from build123d import *

# Parameters (mm, degrees)
SKETCH1_W           = 43
SKETCH1_H           = 43
BOSS_EXTRUDE1_DEPTH = 47
SKETCH2_R           = 10.75
BOSS_EXTRUDE2_DEPTH = 1
SKETCH3_R           = 2.5
BOSS_EXTRUDE3_DEPTH = 20
CHAMFER1_SIZE       = 3
SKETCH4_R           = 1.75
CUT_EXTRUDE2_DEPTH  = 10


with BuildPart() as part:
    # Sketch1 → Boss-Extrude1 (new body)
    with BuildSketch(Plane(origin=(0, 0, 0), x_dir=(1, 0, 0), z_dir=(0, 1, 0))):
        with Locations((21.5, 21.5)):
            Rectangle(SKETCH1_W, SKETCH1_H)
    extrude(amount=BOSS_EXTRUDE1_DEPTH)

    # Sketch2 → Boss-Extrude2 (add)
    with BuildSketch(Plane(origin=(0, 47, 0), x_dir=(1, 0, 0), z_dir=(0, 1, 0))):
        with Locations((21.5, 21.5)):
            Circle(SKETCH2_R)
    extrude(amount=BOSS_EXTRUDE2_DEPTH)

    # Sketch3 → Boss-Extrude3 (add)
    with BuildSketch(Plane(origin=(0, 48, 0), x_dir=(1, 0, 0), z_dir=(0, 1, 0))):
        with Locations((21.5, 21.5)):
            Circle(SKETCH3_R)
    extrude(amount=BOSS_EXTRUDE3_DEPTH)

    # Chamfer1
    chamfer1_edges = [part.edges().sort_by_distance(p)[0] for p in [
        (0, 23.5, -43),
        (43, 23.5, -43),
        (43, 23.5, 0),
        (0, 23.5, 0),
    ]]
    chamfer(chamfer1_edges, length=CHAMFER1_SIZE)

    # Sketch4 → Cut-Extrude2 (cut)
    with BuildSketch(Plane(origin=(0, 47, 0), x_dir=(1, 0, 0), z_dir=(0, 1, 0))):
        with Locations((6, 37)):
            Circle(SKETCH4_R)
        with Locations((6, 6)):
            Circle(SKETCH4_R)
        with Locations((37, 6)):
            Circle(SKETCH4_R)
        with Locations((37, 37)):
            Circle(SKETCH4_R)
    extrude(amount=-CUT_EXTRUDE2_DEPTH, mode=Mode.SUBTRACT)


solid = part.part
Geometry: final body of the model. Coordinates: model frame, mm. A direction names the side the tool comes from. Round coordinates to 2 decimals unless told otherwise and drop trailing zeros. Write each loop counter-clockwise with the first axis right and the second up, starting at its lowest first coordinate (ties: lowest second). Pieces come first, ordered by that corner, then holes. Notation, with made-up numbers: M 33.25,-35 L 82.25,-35 A25 ccw 82.25,-14 Z; hole C -12,10.5 d7. An arc over 180 degrees is marked long. Write item = value, one per line.
Item 1: Section query C-C on z = -37. Return loops of the section in (x, y).
Findings:
outline = M 0,0 L 43,0 L 43,47 L 38.75,47 L 38.75,37 L 35.25,37 L 35.25,47 L 7.75,47 L 7.75,37 L 4.25,37 L 4.25,47 L 0,47 Z
Item 2: Section query B-B on y = 39. Return loops of the section in (x, z).
Findings:
outline = M 0,-40 L 3,-43 L 40,-43 L 43,-40 L 43,-3 L 40,0 L 3,0 L 0,-3 Z; hole C 6,-37 d3.5; hole C 6,-6 d3.5; hole C 37,-37 d3.5; hole C 37,-6 d3.5
Item 3: Pin query (flat end, axial travel): P1, Ø4.5, axis at x = 37, z = -37, coming from the +Y side; P2, Ø1, axis at x = 37.5, z = -6.5, coming from the +Y side; P3, Ø4, axis at x = 22, y = 57.5, coming from the -Z side. Return the tip coordinate at first contact, or that it passes through.
Findings:
P1 = 47
P2 = 37
P3 = -24
Item 4: Section query D-D on y = 54. Return loops of the section in (x, z), then the cut area to 3 significant figures.
Findings:
outline = C 21.5,-21.5 d5
area = 19.6 mm^2
Item 5: Section query A-A on x = 21.5. Return loops of the section in (y, z).
Findings:
outline = M 0,-43 L 47,-43 L 47,-32.25 L 48,-32.25 L 48,-24 L 68,-24 L 68,-19 L 48,-19 L 48,-10.75 L 47,-10.75 L 47,0 L 0,0 Z
Item 6: Material intervals for line 1 along Z through (x, y) = (37, 44.25); line 2 along X through (y, z) = (40, -6); line 3 along Y through (x, z) = (37.5, -34.5), sorted ascending. Write a range as [from, to].
Findings:
line_1 = [-43, -38.75], [-35.25, -7.75], [-4.25, 0]
line_2 = [0, 4.25], [7.75, 35.25], [38.75, 43]
line_3 = [0, 47]
Item 7: Access query for faces 1 (the face through (5.62, 42.07, -35.29)), 2 (the face through (2, 23, -1)). Directions: +Z, -Z, +X, -X, +Y, -Y. A direction counts if a zero-diameter tool reaches every point of the face in a straight line with its end or side. Return the directions, or none.
Findings:
face_1 = +Y
face_2 = +Z, -X, +Y, -Y
Item 8: Pull-direction query (Z, two-part tool) for faces 3 (the face through (5.62, 42.07, -4.29)), 4 (the face through (42, 23, -41)), 5 (the face through (21, 23, 0)), 6 (the face through (6, 37, -37)); classes: pulls with the +Z half, pulls with the -Z half, needs draft (parallel to the pull), parting line crosses it, or undercut.
Findings:
face_3 = undercut
face_4 = pulls with the -Z half
face_5 = pulls with the +Z half
face_6 = undercut
